Can you work these out from the drawing? Everything is in mm from the part's minimum corner. A direction names the side the tool comes from. Coordinates: 2 decimals unless noted, no trailing zeros. Order: outer loops, then holes, each group sorted by start corner. A loop starts at its lowest first (then second) coordinate and runs counter-clockwise, first axis right, second up. Notation, with made-up numbers: (-14, 27) -> (37, 27) arc R19 cw to (37, 52) -> close; hole circle Ø10 at (39, -38.5). An arc over 180 degrees is marked (long way). Return JSON: item names as keys, results as strings. Group by question number.
1) If I drill on probe 1 along X at (y, z) = (24, 46) (1 decimal); probe 2 along X at (y, z) = (51, 45.5); probe 3 along Y at (x, z) = (34.5, 16.5), over which ranges is the centre line in solid material (lowest first)? Write a range as from..to.
2) For the marked faces 1, 2, 3, 4 and 5, which set-ups out of +Z, -Z, +X, -X, +Y, -Y let a thin tool reach every point of the face, with its end or its side?
3) If we section it at B-B, the plane x = 83: Please give me the cut outline in (y, z), then the cut area to 3 significant figures.
4) If we section it at A-A, the plane z = 45: Please give me the cut outline in (x, y).
5) For pin 1 (1 mm diameter, centred on x = 21, y = 42.5, fed in from -Z) (1 decimal); pin 2 (6 mm diameter, centred on x = 55, y = 74, fed in from -Z); pin 3 (4.5 mm diameter, centred on y = 86.5, z = 51, fed in from -X), each with a flat end and sliding along its axis, tell me the tip position at first contact or that it passes through.
6) If we section it at C-C, the plane y = 55: Please give me the cut outline in (x, z).
7) If we section it at D-D, the plane z = 26: Please give me the cut outline in (x, y), then the cut area to 3 significant figures.
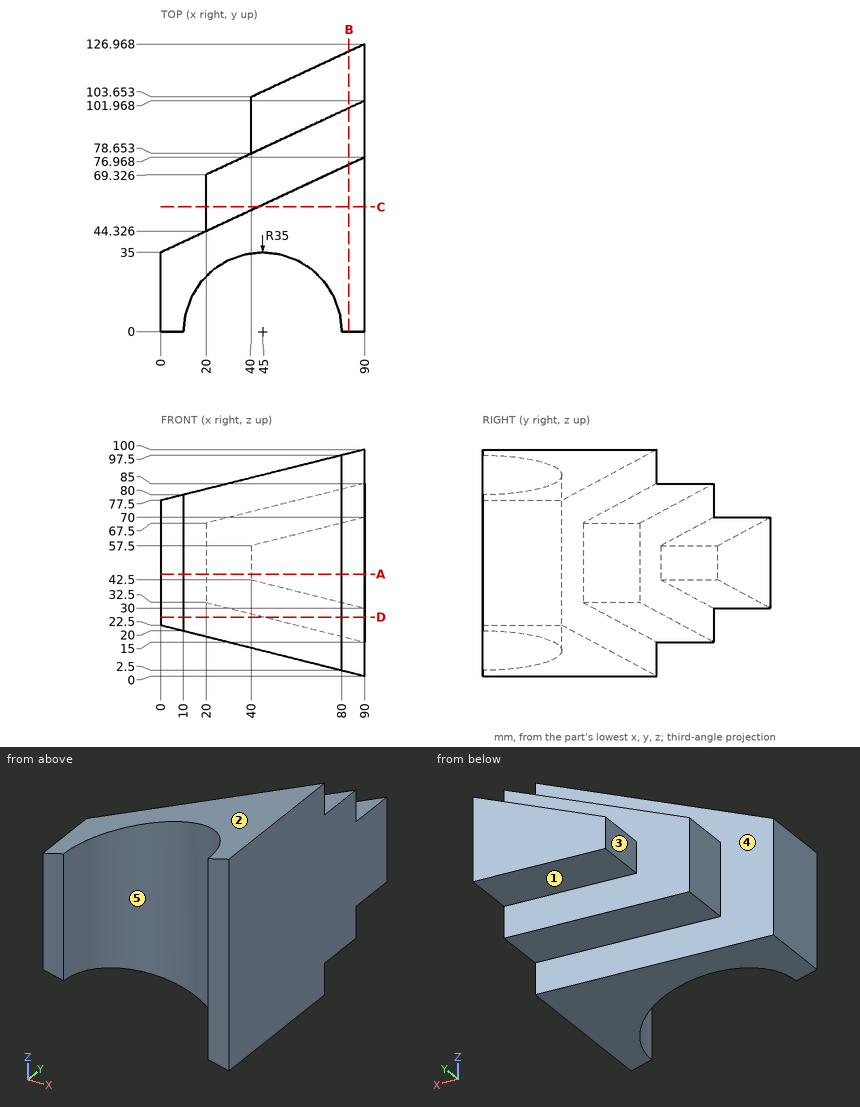
Result sheet:
{
 "1": {"probe 1": "x = 0..19.5, 70.5..90", "probe 2": "x = 20..90", "probe 3": "y = 33.39..51.09"},
 "2": {"face 1": "-Z, -X, +Y", "face 2": "+Z, -X, +Y, -Y", "face 3": "+Z, -Z, -X, +Y", "face 4": "-X, +Y", "face 5": "+Z, -Z, -Y"},
 "3": {"outline": "(0, 1.75) -> (73.7, 1.75) -> (73.7, 16.75) -> (98.7, 16.75) -> (98.7, 31.75) -> (123.7, 31.75) -> (123.7, 68.25) -> (98.7, 68.25) -> (98.7, 83.25) -> (73.7, 83.25) -> (73.7, 98.25) -> (0, 98.25) -> close", "area": "9,690 mm2"},
 "4": {"outline": "(0, 0) -> (10, 0) arc R35 cw to (80, 0) -> (90, 0) -> (90, 126.97) -> (40, 103.65) -> (40, 78.65) -> (20, 69.33) -> (20, 44.33) -> (0, 35) -> close"},
 "5": {"pin 1": "stops at z = 17.1", "pin 2": "stops at z = 23", "pin 3": "stops at x = 40"},
 "6": {"outline": "(20, 32.5) -> (42.89, 26.78) -> (42.89, 11.78) -> (90, 0) -> (90, 100) -> (42.89, 88.22) -> (42.89, 73.22) -> (20, 67.5) -> close"},
 "7": {"outline": "(0, 0) -> (10, 0) arc R35 cw to (80, 0) -> (90, 0) -> (90, 101.97) -> (46, 81.45) -> (46, 56.45) -> (0, 35) -> close", "area": "4,210 mm2"}
}
